Verification items for this drawing (mm, ordinates from the low corner). A direction names the side the tool comes from. Give positions to 0.01 mm unless a question says otherwise; leave off trailing zeros. Loops run counter-clockwise (first coordinate to the right, second up) from the corner with the lowest first, then second, coordinate; pieces in that order, holes last. Notation, with made-up numbers: (74, 79) -> (94, 79) arc R13 cw to (94, 97) -> close; hole circle Ø6 at (-7, 76.5). An arc over 180 degrees is marked (long way). Write each question's results on one line, items separated by ' | '. Start each with the question number.
Item 1: Cross-section at B-B on x = 35. Enter the section's corners in (y, z).
Item 2: Cross-section at C-C on y = 32.5. Enter the section's corners in (x, z).
Item 3: Scan line: line 1 along Z through (x, y) = (19.5, 25.5). Record every from-to range of solid material in increasing order.
Item 4: Cross-section at A-A on z = 21. Enter the section's corners in (x, y), then the cut area to 3 significant figures.
Item 5: Cross-section at D-D on x = 48. Enter the section's corners in (y, z).
Item 6: Access from +Z, -Z, +X, -X, +Y, -Y to the whole of each face (thin tool, end or side, straight path). Record for the marked faces 1 and 2.
Item 7: Gauge pin test, flat ends, axial feed: pin 1 Ø21 at (x, y) = (47, 18) entering from +Z; pin 2 Ø1.6 at (y, z) = (13.5, 29.5) entering from +X; pin 3 Ø8 at (y, z) = (22.5, 33.5) entering from +X; pin 4 Ø12 at (x, z) = (36.5, 35.5) entering from -Y. Record the tip position at first contact, or that the pin passes through.
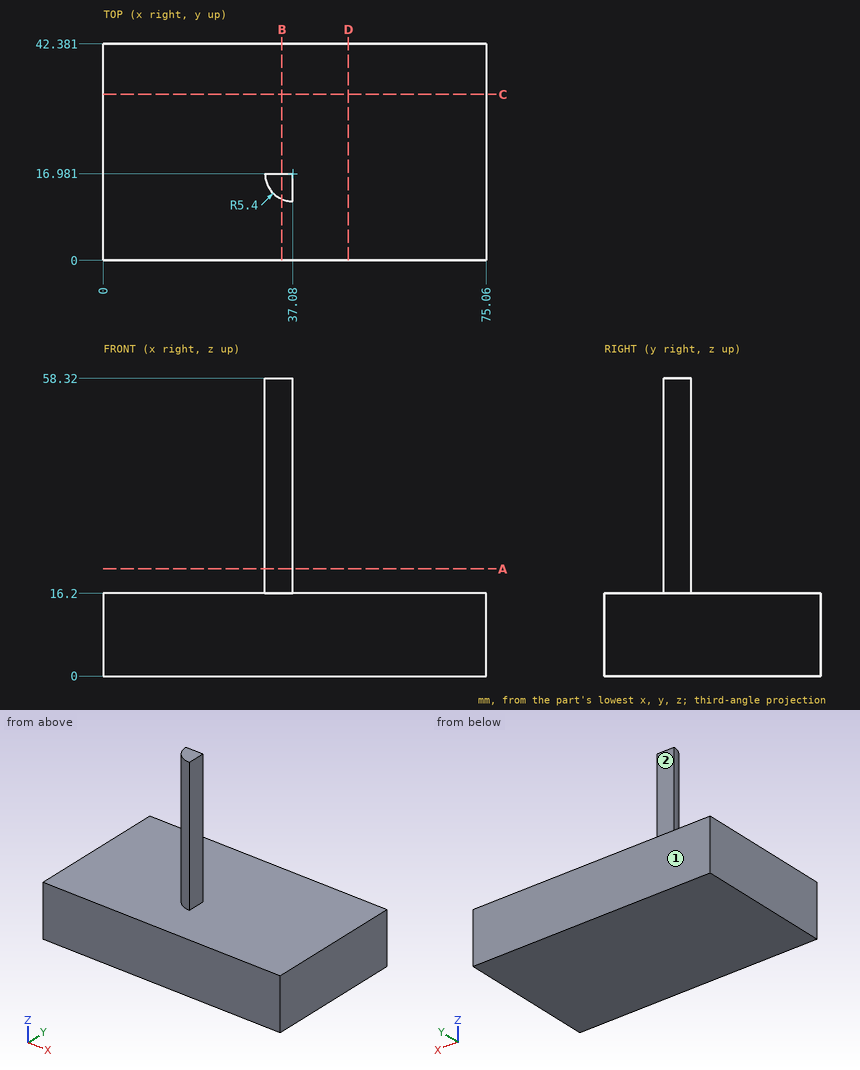
Answer sheet:
1) outline: (0, 0) -> (42.38, 0) -> (42.38, 16.2) -> (16.98, 16.2) -> (16.98, 58.32) -> (12, 58.32) -> (12, 16.2) -> (0, 16.2) -> close
2) outline: (0, 0) -> (75.06, 0) -> (75.06, 16.2) -> (0, 16.2) -> close
3) line 1: z = 0 to 16.2
4) outline: (31.68, 16.98) arc R5.4 ccw to (37.08, 11.58) -> (37.08, 16.98) -> close | area: 22.9 mm²
5) outline: (0, 0) -> (42.38, 0) -> (42.38, 16.2) -> (0, 16.2) -> close
6) face 1: +Z, -Z, +X, -X, +Y | face 2: +Z, +X, -X, +Y
7) pin 1: stops at z = 58.32 | pin 2: stops at x = 37.08 | pin 3: passes through | pin 4: stops at y = 11.58
